Here's how the part is built. I have some questions about the finished solid (model axes, mm). Round coordinates to 2 decimals unless told otherwise and drop trailing zeros. Order: outer loops, then holes, each group sorted by start corner. A loop starts at its lowest first (then second) coordinate and runs counter-clockwise, first axis right, second up. Notation, with made-up numbers: (69.5, -4) - (106.5, -4) arc R22 ccw to (106.5, 35) - close; hole circle Ø1 at (58, 21.25). An arc over 180 degrees is marked (long way). Answer as a JSON object with one key per item and string values.
Autodesk Inventor part; units mm, degrees
ref_plane "YZ Plane" through (0, 0, 0) normal (1, 0, 0) x (0, 1, 0)
ref_plane "XZ Plane" through (0, 0, 0) normal (0, 1, 0) x (-1, 0, 0)
ref_plane "XY Plane" through (0, 0, 0) normal (0, 0, 1) x (1, 0, 0)
sketch "Sketch1" plane through (0, 0, 0) normal (0, 0, 1) x (1, 0, 0)
  line L0 (-29.5, -34.6) -> (29.5, -34.6)
  line L1 (40.1, -24) -> (40.1, 24)
  line L2 (29.5, 34.6) -> (-29.5, 34.6)
  line L3 (-40.1, 24) -> (-40.1, -24)
  line L4 (-40.1, -34.6) -> (40.1, 34.6) construction
  line L5 (40.1, -34.6) -> (-40.1, 34.6) construction
  arc A0 (-29.5, 34.6) -> (-40.1, 24) centre (-29.5, 24) ccw
  arc A1 (-40.1, -24) -> (-29.5, -34.6) centre (-29.5, -24) ccw
  arc A2 (29.5, -34.6) -> (40.1, -24) centre (29.5, -24) ccw
  arc A3 (40.1, 24) -> (29.5, 34.6) centre (29.5, 24) ccw
  point P0 (0, 0)
  dimension "d0" = 69.2
  dimension "d1" = 80.2
  dimension "d2" = 10.6
sketch "Sketch2" plane through (0, 0, 0) normal (0, 1, 0) x (-1, 0, 0)
  line L0 (41.7614, 0.75) -> (40.4386, 0.75)
  arc A0 (40.4386, 0.75) -> (40.4386, -0.75) centre (41.1, 0) ccw
  arc A1 (41.7614, -0.75) -> (41.7614, 0.75) centre (41.1, 0) ccw
  line L1 (41.7614, -0.75) -> (40.4386, -0.75)
  point P0 (0, 0)
  point P1 (40.1, 0)
  point P2 (40.1, 0)
  point P3 (40.1, 0)
  point P4 (41.1, 0.75)
  dimension "d3" = 1.5
  dimension "d4" = 1
sweep "Sweep1" add profiles "Sketch2" path "Sketch1"
properties part number "PayloadGermination_Seal" material "Rubber"
1. Imagine slicing it at A-A (y = 9.5). List the corners of the cut face in (x, z) for me, plus the area to 3 significant figures.
Responses:
{"outline": "(-41.76, -0.75) - (-40.44, -0.75) arc R1 ccw to (-40.44, 0.75) - (-41.76, 0.75) arc R1 ccw to start; (40.44, -0.75) - (41.76, -0.75) arc R1 ccw to (41.76, 0.75) - (40.44, 0.75) arc R1 ccw to start", "area": "5.38 mm2"}
2. Imagine slicing it at C-C (z = -0.2). List the corners of the cut face in (x, y) for me.
Responses:
{"outline": "(-42.08, -24) arc R12.58 ccw to (-29.5, -36.58) - (29.5, -36.58) arc R12.58 ccw to (42.08, -24) - (42.08, 24) arc R12.58 ccw to (29.5, 36.58) - (-29.5, 36.58) arc R12.58 ccw to (-42.08, 24) - close; hole (-40.12, -24) arc R10.62 ccw to (-29.5, -34.62) - (29.5, -34.62) arc R10.62 ccw to (40.12, -24) - (40.12, 24) arc R10.62 ccw to (29.5, 34.62) - (-29.5, 34.62) arc R10.62 ccw to (-40.12, 24) - close"}
3. If I drill on L1, parallel to X at y = 7, z = -0.1; L2, parallel to Y at x = 8, z = -0.05; L3, parallel to X at y = -25, z = 0.15, over which ranges is the centre line in solid material (lowest first)? Write a range as [from, to].
Responses:
{"L1": "[-42.09, -40.11], [40.11, 42.09]", "L2": "[-36.6, -34.6], [34.6, 36.6]", "L3": "[-42.05, -40.06], [40.06, 42.05]"}
4. Imagine slicing it at B-B (x = -23.5). List the corners of the cut face in (y, z) for me.
Responses:
{"outline": "(-36.26, -0.75) - (-34.94, -0.75) arc R1 ccw to (-34.94, 0.75) - (-36.26, 0.75) arc R1 ccw to start; (34.94, -0.75) - (36.26, -0.75) arc R1 ccw to (36.26, 0.75) - (34.94, 0.75) arc R1 ccw to start"}
